```python
from build123d import *
from OCP.BRepFilletAPI import BRepFilletAPI_MakeChamfer

# Parameters (mm, degrees)
SKETCH1_W               = 40
SKETCH1_H               = 40
BOSS_EXTRUDE1_DEPTH     = 8.5
BOSS_EXTRUDE1_TAPER     = 40
SKETCH2_W               = 36
SKETCH2_H               = 36
CUT_EXTRUDE1_DEPTH      = 15
CUT_EXTRUDE1_DRAFT      = -40
SKETCH4_W               = 25.73530627
SKETCH4_H               = 25.73530627
BOSS_EXTRUDE3_DEPTH     = 10
SKETCH5_W               = 22
SKETCH5_H               = 13
CUT_EXTRUDE2_DEPTH      = 31.000000133
CHAMFER2_SIZE           = 12
CHAMFER2_SIZE_2         = 9.89892863
CUT_EXTRUDE3_DEPTH      = 35.154586706
CUT_EXTRUDE3_DEPTH_BACK = 35.154586706
CHAMFER3_SIZE           = 4.3
CHAMFER3_SIZE2          = 7.447818473
CUT_EXTRUDE4_DEPTH      = 35.154586706
CUT_EXTRUDE4_DEPTH_BACK = 35.154586706
SKETCH9_W               = 40.602605658
SKETCH9_H               = 40
BOSS_EXTRUDE4_DEPTH     = 10
BOSS_EXTRUDE4_DRAFT     = -30
SKETCH10_W              = 36.602605658
SKETCH10_H              = 36
CUT_EXTRUDE5_DEPTH      = 10
CUT_EXTRUDE5_DRAFT      = 30


with BuildPart() as part:
    # Sketch1 → Boss-Extrude1 (new body)
    with BuildSketch(Plane(origin=(0, 0, 0), x_dir=(1, 0, 0), z_dir=(0, 1, 0))):
        Rectangle(SKETCH1_W, SKETCH1_H)
    extrude(amount=BOSS_EXTRUDE1_DEPTH, taper=BOSS_EXTRUDE1_TAPER)


with BuildPart() as cut_extrude1_tool:
    # Sketch2 → Cut-Extrude1 (with draft: the straight prism first)
    with BuildSketch(Plane.XZ):
        Rectangle(SKETCH2_W, SKETCH2_H)
    extrude(amount=-CUT_EXTRUDE1_DEPTH)
    # Cut-Extrude1: the draft: its side faces are tilted about the plane it starts from
    cut_extrude1_sides = [cut_extrude1_tool.faces().sort_by_distance(p)[0] for p in [
        (0, 7.5, -18),
        (18, 7.5, 0),
        (0, 7.5, 18),
        (-18, 7.5, 0),
    ]]
    draft(cut_extrude1_sides, Plane.XZ, CUT_EXTRUDE1_DRAFT)


with BuildPart() as part_1:
    add(part.part)

    # Cut-Extrude1: cut by cut_extrude1_tool
    add(cut_extrude1_tool.part, mode=Mode.SUBTRACT)

    # Sketch4 → Boss-Extrude3 (add)
    with BuildSketch(Plane(origin=(0, 8.5, 0), x_dir=(1, 0, 0), z_dir=(0, 1, 0))):
        Rectangle(SKETCH4_W, SKETCH4_H)
    extrude(amount=BOSS_EXTRUDE3_DEPTH)

    # Sketch5 → Cut-Extrude2 (cut, through all)
    with BuildSketch(Plane.XZ.offset(-8.5)):
        Rectangle(SKETCH5_W, SKETCH5_H)
    extrude(amount=-CUT_EXTRUDE2_DEPTH, mode=Mode.SUBTRACT)

    # Chamfer2
    # the kernel refuses this chamfer: 12, 9.89892863 mm, written as the material it adds along each edge
    with BuildSketch(Plane(origin=(12.867653135, 8.5, 44.011128682), x_dir=(0.6427876096865404, -0.7660444431189772, 0), z_dir=(0, 0, -1))) as chamfer2_piece_1_section:
        Polygon((CHAMFER2_SIZE, 0), (-CHAMFER2_SIZE_2 * 0.766044443108, -CHAMFER2_SIZE_2 * 0.642787609677), (0, 0), align=None)
    chamfer2_piece_1 = extrude(amount=88.022257365, mode=Mode.PRIVATE)
    chamfer2_piece_1 = split(chamfer2_piece_1, bisect_by=Plane(origin=(12.867653135, 0, 44.011128682), z_dir=(0, 1, 0)), keep=Keep.TOP, mode=Mode.PRIVATE)
    chamfer2_piece_1 = split(chamfer2_piece_1, bisect_by=Plane(origin=(12.867653135, -0.927920344, 20.676206983), z_dir=(0, -0.37460659341591307, -0.927183854566787)), keep=Keep.TOP, mode=Mode.PRIVATE)
    chamfer2_piece_1 = split(chamfer2_piece_1, bisect_by=Plane(origin=(12.867653135, 29.644778588, -8.32403482), z_dir=(0, -0.3746065934159128, 0.9271838545667871)), keep=Keep.TOP, mode=Mode.PRIVATE)
    add(chamfer2_piece_1)
    with BuildSketch(Plane(origin=(-12.867653135, 8.5, -44.011128682), x_dir=(-0.6427876096865406, -0.766044443118977, 0), z_dir=(0, 0, 1))) as chamfer2_piece_2_section:
        Polygon((CHAMFER2_SIZE, 0), (-CHAMFER2_SIZE_2 * 0.766044443108, -CHAMFER2_SIZE_2 * 0.642787609677), (0, 0), align=None)
    chamfer2_piece_2 = extrude(amount=88.022257365, mode=Mode.PRIVATE)
    chamfer2_piece_2 = split(chamfer2_piece_2, bisect_by=Plane(origin=(-12.867653135, 0, -44.011128682), z_dir=(0, 1, 0)), keep=Keep.TOP, mode=Mode.PRIVATE)
    chamfer2_piece_2 = split(chamfer2_piece_2, bisect_by=Plane(origin=(-12.867653135, -0.927920344, -20.676206983), z_dir=(0, -0.3746065934159128, 0.9271838545667871)), keep=Keep.TOP, mode=Mode.PRIVATE)
    chamfer2_piece_2 = split(chamfer2_piece_2, bisect_by=Plane(origin=(-12.867653135, 29.644778588, 8.32403482), z_dir=(0, -0.37460659341591307, -0.927183854566787)), keep=Keep.TOP, mode=Mode.PRIVATE)
    add(chamfer2_piece_2)
    with BuildSketch(Plane(origin=(-44.011128682, 8.5, 12.867653135), x_dir=(0, -0.766044443118977, 0.6427876096865405), z_dir=(1, 0, 0))) as chamfer2_piece_3_section:
        Polygon((CHAMFER2_SIZE, 0), (-CHAMFER2_SIZE_2 * 0.766044443108, -CHAMFER2_SIZE_2 * 0.642787609677), (0, 0), align=None)
    chamfer2_piece_3 = extrude(amount=88.022257365, mode=Mode.PRIVATE)
    chamfer2_piece_3 = split(chamfer2_piece_3, bisect_by=Plane(origin=(-44.011128682, 0, 12.867653135), z_dir=(0, 1, 0)), keep=Keep.TOP, mode=Mode.PRIVATE)
    chamfer2_piece_3 = split(chamfer2_piece_3, bisect_by=Plane(origin=(-20.676206983, -0.927920344, 12.867653135), z_dir=(0.927183854566787, -0.37460659341591307, 0)), keep=Keep.TOP, mode=Mode.PRIVATE)
    chamfer2_piece_3 = split(chamfer2_piece_3, bisect_by=Plane(origin=(8.32403482, 29.644778588, 12.867653135), z_dir=(-0.9271838545667872, -0.37460659341591274, 0)), keep=Keep.TOP, mode=Mode.PRIVATE)
    add(chamfer2_piece_3)
    with BuildSketch(Plane(origin=(44.011128682, 8.5, -12.867653135), x_dir=(0, -0.766044443118977, -0.6427876096865405), z_dir=(-1, 0, 0))) as chamfer2_piece_4_section:
        Polygon((CHAMFER2_SIZE, 0), (-CHAMFER2_SIZE_2 * 0.766044443108, -CHAMFER2_SIZE_2 * 0.642787609677), (0, 0), align=None)
    chamfer2_piece_4 = extrude(amount=88.022257365, mode=Mode.PRIVATE)
    chamfer2_piece_4 = split(chamfer2_piece_4, bisect_by=Plane(origin=(44.011128682, 0, -12.867653135), z_dir=(0, 1, 0)), keep=Keep.TOP, mode=Mode.PRIVATE)
    chamfer2_piece_4 = split(chamfer2_piece_4, bisect_by=Plane(origin=(-8.32403482, 29.644778588, -12.867653135), z_dir=(0.927183854566787, -0.37460659341591307, 0)), keep=Keep.TOP, mode=Mode.PRIVATE)
    chamfer2_piece_4 = split(chamfer2_piece_4, bisect_by=Plane(origin=(20.676206983, -0.927920344, -12.867653135), z_dir=(-0.9271838545667872, -0.37460659341591274, 0)), keep=Keep.TOP, mode=Mode.PRIVATE)
    add(chamfer2_piece_4)

    # Sketch7 → Cut-Extrude3 (cut, two sides: drawn at the far end of the back side and taken through both)
    with BuildSketch(Plane(origin=(0, 0, 0), x_dir=(0, 0, -1), z_dir=(1, 0, 0)).offset(-CUT_EXTRUDE3_DEPTH_BACK)):
        Polygon((-20, 0), (-24.78585356, 0), (-24.78585356, 18.532984169), (-10.14, 18.5), align=None)
    extrude(amount=CUT_EXTRUDE3_DEPTH + CUT_EXTRUDE3_DEPTH_BACK, mode=Mode.SUBTRACT)

    # Chamfer3: one chamfer whose edges measure the first distance from different faces: ONE call of the kernel's chamfer builder (chamfer() names one face for all edges)
    chamfer3_edges_1 = [part_1.edges().sort_by_distance(p)[0] for p in [
        (0, 8.5, 6.5),
    ]]
    chamfer3_side_1 = [part_1.faces().sort_by_distance(p)[0] for p in [
        (0, 8.5, 8.683826567),
    ]]
    chamfer3_edges_2 = [part_1.edges().sort_by_distance(p)[0] for p in [
        (0, 8.5, -6.5),
    ]]
    chamfer3_side_2 = [part_1.faces().sort_by_distance(p)[0] for p in [
        (0, 8.5, -8.683826567),
    ]]
    chamfer3 = BRepFilletAPI_MakeChamfer(part_1.part.solid().wrapped)
    for e in chamfer3_edges_1:
        chamfer3.Add(CHAMFER3_SIZE, CHAMFER3_SIZE2, e.wrapped, chamfer3_side_1[0].wrapped)  # the first distance lies on this face
    for e in chamfer3_edges_2:
        chamfer3.Add(CHAMFER3_SIZE, CHAMFER3_SIZE2, e.wrapped, chamfer3_side_2[0].wrapped)  # the first distance lies on this face
    add(Compound.cast(chamfer3.Shape()), mode=Mode.REPLACE)

    # Sketch8 → Cut-Extrude4 (cut, two sides: drawn at the far end of the back side and taken through both)
    with BuildSketch(Plane(origin=(0, 0, 0), x_dir=(0, 0, -1), z_dir=(1, 0, 0)).offset(-CUT_EXTRUDE4_DEPTH_BACK)):
        Polygon((7.63, 18.5), (12.867653135, 18.5), (21.160182577, 0), (20, 0), align=None)
    extrude(amount=CUT_EXTRUDE4_DEPTH + CUT_EXTRUDE4_DEPTH_BACK, mode=Mode.SUBTRACT)


with BuildPart() as boss_extrude4_tool:
    # Sketch9 → Boss-Extrude4 (with draft: the straight prism first)
    with BuildSketch(Plane.XZ):
        Rectangle(SKETCH9_W, SKETCH9_H)
    extrude(amount=BOSS_EXTRUDE4_DEPTH)
    # Boss-Extrude4: the draft: its side faces are tilted about the plane it starts from
    boss_extrude4_sides = [boss_extrude4_tool.faces().sort_by_distance(p)[0] for p in [
        (0, -5, -20),
        (20.301302829, -5, 0),
        (0, -5, 20),
        (-20.301302829, -5, 0),
    ]]
    draft(boss_extrude4_sides, Plane.XZ, BOSS_EXTRUDE4_DRAFT)


with BuildPart() as part_2:
    add(part_1.part)

    # Boss-Extrude4: add boss_extrude4_tool
    add(boss_extrude4_tool.part)


with BuildPart() as cut_extrude5_tool:
    # Sketch10 → Cut-Extrude5 (with draft: the straight prism first)
    with BuildSketch(Plane(origin=(0, 0, 0), x_dir=(1, 0, 0), z_dir=(0, 1, 0))):
        Rectangle(SKETCH10_W, SKETCH10_H)
    extrude(amount=-CUT_EXTRUDE5_DEPTH)
    # Cut-Extrude5: the draft: its side faces are tilted about the plane it starts from
    cut_extrude5_sides = [cut_extrude5_tool.faces().sort_by_distance(p)[0] for p in [
        (0, -5, 18),
        (18.301302829, -5, 0),
        (0, -5, -18),
        (-18.301302829, -5, 0),
    ]]
    draft(cut_extrude5_sides, Plane(origin=(0, 0, 0), x_dir=(1, 0, 0), z_dir=(0, 1, 0)), CUT_EXTRUDE5_DRAFT)


with BuildPart() as part_3:
    add(part_2.part)

    # Cut-Extrude5: cut by cut_extrude5_tool
    add(cut_extrude5_tool.part, mode=Mode.SUBTRACT)


solid = part_3.part
```
Can you work these out from the model? Positions are in its coordinate system, mm. A direction names the side the tool comes from. Coordinates: 2 decimals unless noted, no trailing zeros. Loops run counter-clockwise (first coordinate to the right, second up) from the corner with the lowest first, then second, coordinate; pieces in that order, holes last. Notation, with made-up numbers: M -30.75,85.5 L 6.25,85.5 A15 cw 6.25,99.5 Z; hole C 60.5,48 d11. An arc over 180 degrees is marked long. Put each result on its own line as item: value. Start each with the question number.
(1) We'd pull the mould along Z, two halves only. Please class faces 4 (the face through (-0.365, -4.93, -22.846)), 5 (the face through (0, 17, -6.5)), 6 (the face through (-0.28, 9.38, 15)), 7 (the face through (0, 18.5, 7)): +Z half, -Z half, draft (parallel to the pull), parting line (faces both ways), or undercut.
(2) Imagine slicing it at B-B on z = -17. List the corners of the cut face in (x, y) for me, and give its area (3 significant figures).
(3) Imagine slicing it at A-A on y = 5.25. List the corners of the cut face in (x, z) for me, and give its area (3 significant figures).
(4) Will these pins go through, and if not, where does the flat tip stop? pin 1 Ø12 at (y, z) = (3.5, 5) entering from -X; pin 2 Ø11 at (y, z) = (13, 3) entering from -X; pin 3 Ø4 at (x, z) = (-3, -5) entering from -Y.
(5) Imagine slicing it at D-D on y = 9.75. List the corners of the cut face in (x, z) for me.
(6) Which directions (+Z, -Z, +X, -X, +Y, -Y) give clear straight access to the entire face, cutting with the end or side of a thin tool? Please do faces 1 (the face through (11, 13, 0)), 2 (the face through (-0.152, 11.449, -9.098)), 3 (the face through (-17.46, 7.03, -0.28)).
(7) Imagine slicing it at C-C on x = 19. List the corners of the cut face in (y, z) for me, and give its area (3 significant figures).
(8) I need wall thicknesses on probe 1 along Z at (x, y) = (15.5, -1.25); probe 2 along Z at (x, y) = (-3.5, 6); probe 3 along X at (y, z) = (0.25, -15.5). Which ranges of each line are inside material? Lowest first, please.
Worked answers:
1. face 4: -Z half
1. face 5: undercut
1. face 6: +Z half
1. face 7: draft
2. outline: M -26.07,-10 L -24.07,-10 L -18.3,0 L -18,0 L -17,1.19 L 17,1.19 L 18,0 L 18.3,0 L 24.07,-10 L 26.07,-10 L 20.3,0 L 18.49,4.49 L -18.49,4.49 L -20.3,0 Z
2. area: 172 mm2
3. outline: M -18.18,-16.49 L 18.18,-16.49 L 18.18,17.2 L -18.18,17.2 Z; hole M -13.59,-13.59 L 13.59,-13.59 L 13.59,13.59 L -13.59,13.59 Z
3. area: 486 mm2
4. pin 1: stops at x = -21.74
4. pin 2: stops at x = -17.27
4. pin 3: stops at y = 15.08
5. outline: M -16.36,-13.48 L 16.36,-13.48 L 16.36,14.8 L -16.36,14.8 Z; hole M -11,-6.5 L -9.82,-6.5 L -9.82,-10.08 L 9.82,-10.08 L 9.82,-6.5 L 11,-6.5 L 11,6.5 L 9.82,6.5 L 9.82,10.08 L -9.82,10.08 L -9.82,6.5 L -11,6.5 Z
6. face 1: +Y
6. face 2: -Y
6. face 3: +Z, -Z, -X, +Y
7. outline: M -10,-25.77 L 0,-20 L 3.22,-17.85 L 3.22,18.28 L 0,20 L -10,25.77 L -10,23.77 L -1.21,18.7 L -1.21,-18.7 L -10,-23.77 Z
7. area: 207 mm2
8. probe 1: z = -20.72 to -18.72, 18.72 to 20.72
8. probe 2: z = -15.99 to -12.97, 12.97 to 16.8
8. probe 3: x = -20.2 to -17.79, 17.79 to 20.2
